Job drawing, mm, ordinate dimensions from the low corner. One solid piece. A direction names the side the tool comes from. Give positions to 0.01 mm unless a question says otherwise; leave off trailing zeros. Loops run counter-clockwise (first coordinate to the right, second up) from the corner with the lowest first, then second, coordinate; pieces in that order, holes last. Notation, with made-up numbers: (-5, -8) -> (0, -8) arc R10 ccw to (0, 10) -> close; hole circle Ø9 at (-5.75, 79). An arc over 180 degrees is marked (long way). Answer as a JSON object with one key per item and string values. Group by question number.
Q1. Band-saw the part on A-A, the plane z = 25. Write the cut outline in (x, y), plus the area to 3 significant figures.
Q2. Drop flat-ended pins along their axis: pin 1 (1 mm diameter, centred on x = 24.5, z = 14.5, fed in from -Y); pin 2 (11 mm diameter, centred on y = 6.5, z = 24.5, fed in from +X); pin 3 (3 mm diameter, centred on x = 33.5, y = 7.5, fed in from -Z) (1 decimal). Give the stop position or say it passes through.
Q3. Band-saw the part on B-B, the plane y = 16.25. Count the separate pieces of the cut face and the enclosed holes in it, plus the area to 3 significant figures.
Q4. Two-plate mould, pull along Z, no slides. Class the marked faces 1, 2 and 3: pulls with the +Z half, pulls with the -Z half, needs draft (parallel to the pull), parting line crosses it, or undercut.
Q5. Band-saw the part on C-C, the plane y = 2. Write the cut outline in (x, z) (1 decimal), plus the area to 3 significant figures.
Q6. Wall check: probe 1 along Z at (x, y) = (32, 9.5); probe 2 along Z at (x, y) = (25.5, 5.75) (1 decimal); probe 3 along X at (y, z) = (16, 13.5). Give the ranges that are in metal, low to high. Write a range as from..to.
Q7. Tool access for the marked faces 4, 5, 6 and 7: list every direction of +Z, -Z, +X, -X, +Y, -Y with a clear straight run to the whole face (end or side of a thin tool).
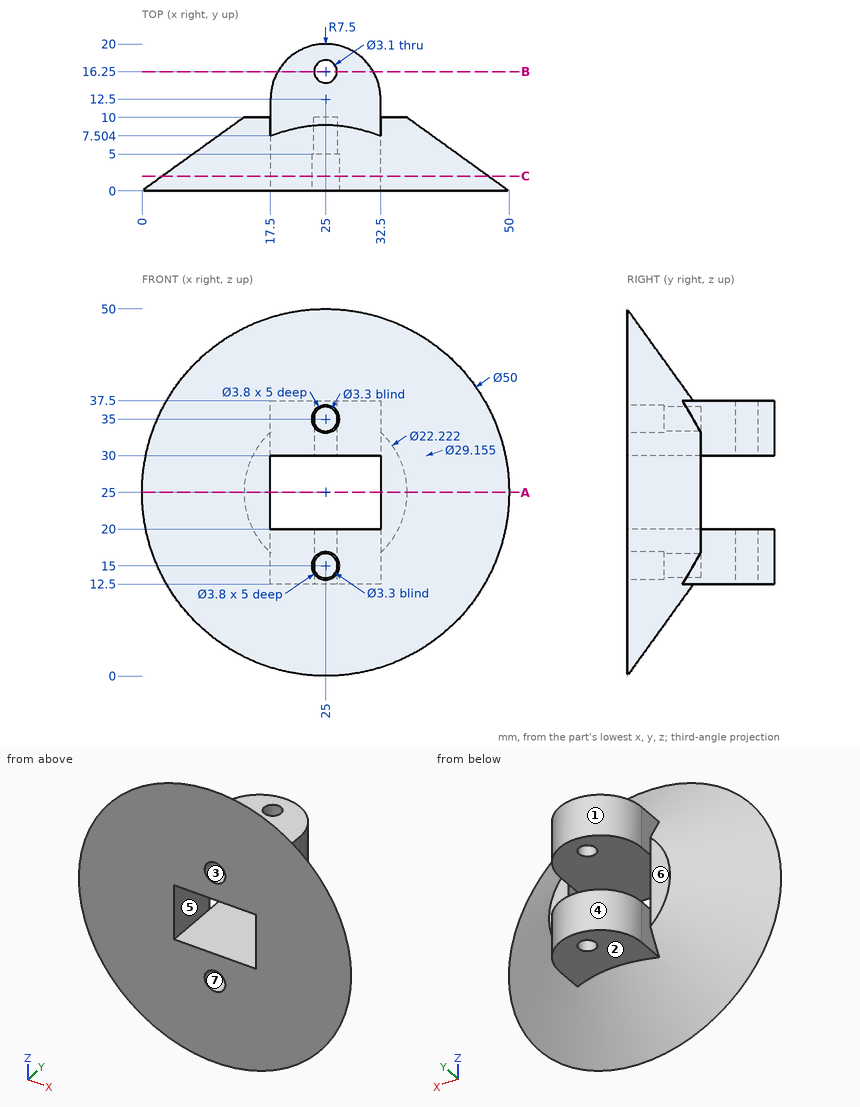
Worked answers:
{
 "1": {"outline": "(0, 0) -> (17.5, 0) -> (17.5, 10) -> (13.89, 10) -> close; (32.5, 0) -> (50, 0) -> (36.11, 10) -> (32.5, 10) -> close", "area": "211 mm2"},
 "2": {"pin 1": "y = 10", "pin 2": "x = 48.61", "pin 3": "z = 10.5"},
 "3": {"separate pieces": "4", "enclosed holes": "0", "area": "148 mm2"},
 "4": {"face 1": "needs draft", "face 2": "pulls with the -Z half", "face 3": "undercut"},
 "5": {"outline": "circle Ø44.4 at (25, 25); hole (17.5, 20) -> (32.5, 20) -> (32.5, 30) -> (17.5, 30) -> close; hole circle Ø3.8 at (25, 15); hole circle Ø3.8 at (25, 35)", "area": "1,380 mm2"},
 "6": {"probe 1": "12.5..20, 30..37.5", "probe 2": "8..13.4, 16.6..20, 30..33.4, 36.6..42", "probe 3": "18.37..23.47, 26.53..31.63"},
 "7": {"face 4": "+Z, -Z, +Y", "face 5": "+Y, -Y", "face 6": "+Z, -Z, -X, +Y", "face 7": "-Y"}
}
